Verification items for the finished model (mm, model axes). Face numbers are marked on the shaded views. A direction names the side the tool comes from. Coordinates: 2 decimals unless noted, no trailing zeros. Order: outer loops, then holes, each group sorted by start corner. A loop starts at its lowest first (then second) coordinate and runs counter-clockwise, first axis right, second up. Notation, with made-up numbers: M -36,51 L 13,51 A29 ccw 13,76 Z; hole C -12.5,30.5 d9. An arc over 180 degrees is marked long. Return JSON: item names as keys, results as strings. Group by question number.
Q1. Thickness scan on probe 1 along X at (y, z) = (-2, 11); probe 2 along Z at (x, y) = (34, -14.5); probe 3 along Y at (x, z) = (9, 61). Record the ranges inside material, lowest first.
Q2. Access from +Z, -Z, +X, -X, +Y, -Y to the whole of each face (thin tool, end or side, straight path). Record for the marked faces 1, 2 and 3.
Q3. Section check A-A, the plane x = 35. Enter the section's corners in (y, z), then the cut area to 3 significant figures.
Q4. Section check B-B, the plane y = -6. Enter the section's corners in (x, z).
Q5. Go/stop test with flat-tipped pins: pin 1 Ø1.8 at (x, z) = (0, 23.5) entering from -Y; pin 2 Ø3 at (x, z) = (20, 66.5) entering from +Y; pin 3 Ø9.5 at (x, y) = (21, -11) entering from -Z. Record where each tip stops, or that it passes through.
from build123d import *

# Parameters (mm, degrees)
SKETCH1_W           = 6
SKETCH1_H           = 10
BOSS_EXTRUDE1_DEPTH = 70
SKETCH2_W           = 6
SKETCH2_H           = 10
BOSS_EXTRUDE2_DEPTH = 12
SKETCH3_W           = 10
SKETCH3_H           = 10
BOSS_EXTRUDE3_DEPTH = 40


with BuildPart() as part:
    # Sketch1 → Boss-Extrude1 (new body)
    with BuildSketch(Plane.XY):
        Rectangle(SKETCH1_W, SKETCH1_H)
    extrude(amount=BOSS_EXTRUDE1_DEPTH)

    # Sketch2 → Boss-Extrude2 (add)
    with BuildSketch(Plane.XZ.offset(5)):
        with Locations((0, 65)):
            Rectangle(SKETCH2_W, SKETCH2_H)
    extrude(amount=BOSS_EXTRUDE2_DEPTH)

    # Sketch3 → Boss-Extrude3 (add)
    with BuildSketch(Plane(origin=(3, 0, 0), x_dir=(0, 0, -1), z_dir=(1, 0, 0))):
        with Locations((-65, -12)):
            Rectangle(SKETCH3_W, SKETCH3_H)
    extrude(amount=BOSS_EXTRUDE3_DEPTH)


solid = part.part
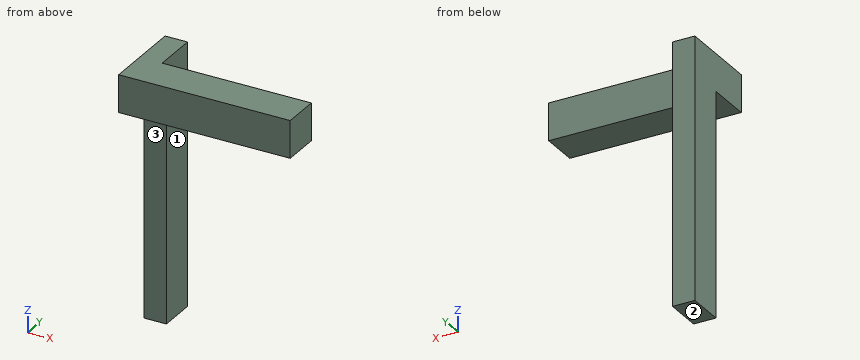
Numbers:
{
 "1": {"probe 1": "x = -3 to 3", "probe 2": "z = 60 to 70", "probe 3": "y = -17 to -7"},
 "2": {"face 1": "+Z, -Z, +X, +Y", "face 2": "-Z, +X, -X, +Y, -Y", "face 3": "-Z, +X, -X, -Y"},
 "3": {"outline": "M -17,60 L -7,60 L -7,70 L -17,70 Z", "area": "100 mm2"},
 "4": {"outline": "M -3,60 L 3,60 L 3,70 L -3,70 Z"},
 "5": {"pin 1": "stops at y = -5", "pin 2": "stops at y = -7", "pin 3": "stops at z = 60"}
}
